from build123d import *

# Parameters (mm, degrees)
EXTRUDE_1_DEPTH     = 65
SKETCH_4_R          = 2.25
CUT_EXTRUDE_2_DEPTH = 44
CUT_EXTRUDE_START   = -5
SKETCH_5_R          = 3.75
CUT_EXTRUDE_3_DEPTH = 44
EXTRUDE_2_DEPTH     = 5
EXTRUDE_4_DEPTH     = 8
SKETCH_9_R          = 2.3
CUT_EXTRUDE_4_DEPTH = 3.5
CUT_EXTRUDE_6_DEPTH = 14
CUT_EXTRUDE_7_DEPTH = 5


with BuildPart() as part:
    # ｽｹｯﾁ1 → ﾎﾞｽ - 押し出し1 (new body)
    with BuildSketch(Plane.XY):
        Polygon((0, 0), (9.641814145, 11.490666647), (-1.848852501, 21.132480792), (1.365085547, 24.962703008), (65.946194887, 24.962703008), (65.946194887, 19.962703008), (3.830222216, -3.213938048), align=None)
    extrude(amount=EXTRUDE_1_DEPTH)

    # ｽｹｯﾁ4 → ｶｯﾄ - 押し出し2 (cut)
    with BuildSketch(Plane(origin=(9.641814145, 11.490666647, 0), x_dir=(-0.766044443, 0.64278761, 0), z_dir=(-0.64278761, -0.766044443, 0))):
        with Locations((7.5, -12.5)):
            Circle(SKETCH_4_R)
        with Locations((7.5, -57.5)):
            Circle(SKETCH_4_R)
    extrude(amount=-CUT_EXTRUDE_2_DEPTH, mode=Mode.SUBTRACT)

    # ｽｹｯﾁ5 → ｶｯﾄ - 押し出し3 (cut)
    with BuildSketch(Plane(origin=(9.641814145, 11.490666647, 0), x_dir=(-0.766044443, 0.64278761, 0), z_dir=(-0.64278761, -0.766044443, 0)).offset(CUT_EXTRUDE_START)):
        with Locations((7.5, -57.5)):
            Circle(SKETCH_5_R)
        with Locations((7.5, -12.5)):
            Circle(SKETCH_5_R)
    extrude(amount=-CUT_EXTRUDE_3_DEPTH, mode=Mode.SUBTRACT)

    # ｽｹｯﾁ6 → ﾎﾞｽ - 押し出し2 (add)
    with BuildSketch(Plane.XY):
        Polygon((0, 0), (3.830222216, -3.213938048), (65.946194887, 19.962703008), (65.946194887, 34.162703008), (9.084802154, 34.162703008), (-1.848852501, 21.132480792), (9.641814145, 11.490666647), align=None)
    extrude(amount=-EXTRUDE_2_DEPTH)

    # ｽｹｯﾁ8 → ﾎﾞｽ - 押し出し4 (add)
    with BuildSketch(Plane.XY):
        Polygon((65.946194887, 34.162703008), (65.946194887, 29.162703008), (4.889303998, 29.162703008), (9.084802154, 34.162703008), align=None)
    extrude(amount=EXTRUDE_4_DEPTH)

    # ｽｹｯﾁ9 → ｶｯﾄ - 押し出し4 (cut)
    with BuildSketch(Plane(origin=(0, 24.962703008, 0), x_dir=(1, 0, 0), z_dir=(0, 1, 0))):
        with Locations((16.255085547, -35)):
            Circle(SKETCH_9_R)
    extrude(amount=-CUT_EXTRUDE_4_DEPTH, mode=Mode.SUBTRACT)

    # ｽｹｯﾁ11 → ｶｯﾄ - 押し出し6 (cut, through all)
    with BuildSketch(Plane.XY.offset(8)):
        Polygon((1.365085547, 24.962703008), (20.364802154, 24.962703008), (20.364802154, 34.162703008), (9.084802154, 34.162703008), align=None)
    extrude(amount=-CUT_EXTRUDE_6_DEPTH, mode=Mode.SUBTRACT)

    # ｽｹｯﾁ12 → ｶｯﾄ - 押し出し7 (cut)
    with BuildSketch(Plane(origin=(65.946194887, 0, 0), x_dir=(0, 0, -1), z_dir=(1, 0, 0))):
        Polygon((0, 24.962703008), (5, 24.962703008), (5, 34.162703008), (-8, 34.162703008), (-8, 29.162703008), (0, 29.162703008), align=None)
    extrude(amount=-CUT_EXTRUDE_7_DEPTH, mode=Mode.SUBTRACT)


solid = part.part
Could you check a few things on this model? Use its own coordinates, in mm. A direction names the side the tool comes from. Give positions to 0.01 mm unless a question says otherwise; leave off trailing zeros. Loops run counter-clockwise (first coordinate to the right, second up) from the corner with the lowest first, then second, coordinate; pieces in that order, holes last. Notation, with made-up numbers: M -38.75,-22 L -18.75,-22 A21 ccw -18.75,-12 Z; hole C 67,21 d3. An arc over 180 degrees is marked long. Answer as a JSON object with one key per item and string values.
Q1. Suppose I cut it at B-B, the plane x = 41. List the corners of the cut face in (y, z) for me.
Values found:
{"outline": "M 10.65,-5 L 34.16,-5 L 34.16,8 L 29.16,8 L 29.16,0 L 24.96,0 L 24.96,65 L 10.65,65 Z"}
Q2. Suppose I cut it at C-C, the plane y = 26. List the corners of the cut face in (x, z) for me, plus the area to 3 significant figures.
Values found:
{"outline": "M 20.36,-5 L 60.95,-5 L 60.95,0 L 20.36,0 Z", "area": "203 mm²"}
Q3. Suppose I cut it at A-A, the plane z = 25. List the corners of the cut face in (x, y) for me, plus the area to 3 significant figures.
Values found:
{"outline": "M -1.85,21.13 L 9.64,11.49 L 0,0 L 3.83,-3.21 L 65.95,19.96 L 65.95,24.96 L 1.37,24.96 Z", "area": "1,040 mm²"}
Q4. Suppose I cut it at D-D, the plane z = 35. List the corners of the cut face in (x, y) for me, plus the area to 3 significant figures.
Values found:
{"outline": "M -1.85,21.13 L 9.64,11.49 L 0,0 L 3.83,-3.21 L 65.95,19.96 L 65.95,24.96 L 18.56,24.96 L 18.56,21.46 L 13.96,21.46 L 13.96,24.96 L 1.37,24.96 Z", "area": "1,020 mm²"}
Q5. For faces 1 (the flat face through (41, 32, 8)), 2 (the flat face through (16, 21.463, 35)), 3 (the flat face through (41, 29.163, 4)), 4 (the flat face through (4.89, 5.83, 30.49)), 5 (the flat face through (20.365, 31, 0)), which set-ups out of +Z, -Z, +X, -X, +Y, -Y let a thin tool reach every point of the face, with its end or its side?
Values found:
{"face 1": "+Z, +X, -X, +Y", "face 2": "+Y", "face 3": "+Z, +X, -X", "face 4": "+Z, -Z, -X", "face 5": "+Z, -Z, -X, +Y"}
Q6. If I drill on probe 1 along Y at (x, z) = (4, 21.5); probe 2 along Z at (x, y) = (32.5, 27); probe 3 along X at (y, z) = (23, 35), over which ranges is the centre line in solid material (lowest first)? Write a range as [from, to].
Values found:
{"probe 1": "y = [-3.15, 4.77], [16.22, 24.96]", "probe 2": "z = [-5, 0]", "probe 3": "x = [-0.28, 13.96], [18.56, 65.95]"}
Q7. If we mould it in two halves opening along Y, with no side actions, what happens to faces 6 (the flat face through (1.888, -1.584, 30.49)), 7 (the flat face through (40, 34.163, 1)), 8 (the flat face through (7.15, 20.11, 59.95))? For each: pulls with the +Y half, pulls with the -Y half, needs draft (parallel to the pull), parting line crosses it, or undercut.
Values found:
{"face 6": "pulls with the -Y half", "face 7": "pulls with the +Y half", "face 8": "undercut"}
Q8. For P1, Ø2, axis at x = 38.5, y = 27, coming from the +Z side; P2, Ø2, axis at y = 3, z = 40.5, coming from the -X side; P3, Ø3, axis at x = 38, z = 49, coming from the -Y side, each with a flat end and sliding along its axis, tell me the tip position at first contact or that it passes through.
Values found:
{"P1": "stops at z = 0", "P2": "stops at x = 1.68", "P3": "stops at y = 8.98"}
